Verification items for the finished model (mm, model axes). A direction names the side the tool comes from. Round coordinates to 2 decimals unless told otherwise and drop trailing zeros. Order: outer loops, then holes, each group sorted by start corner. A loop starts at its lowest first (then second) coordinate and runs counter-clockwise, first axis right, second up. Notation, with made-up numbers: (87, 42.5) -> (130, 42.5) arc R30 ccw to (130, 71.5) -> close; hole circle Ø10 at (26, 61). An arc over 180 degrees is marked (long way). Return JSON: item names as keys, results as strings. Group by question number.
1) Tool access check on faces 1 (the flat face through (-5.4, -3.2, 0)), 2 (the flat face through (5.4, -3.2, 0)), 3 (the flat face through (-5.4, 3, 0)). Record the directions out of +Z, -Z, +X, -X, +Y, -Y that give a thin tool (end or side, any length) a straight path to the whole face; none if there is none.
2) Depth check by flat-ended pin: pin 1 (2 mm diameter, centred on x = 2, z = -9.5, fed in from +Y); pin 2 (1 mm diameter, centred on x = 3.5, z = 4, fed in from +Y); pin 3 (2.5 mm diameter, centred on x = -2, y = -1, fed in from -Z). Enter the tip coordinate at first touch or a pass-through.
3) Section check A-A on z = 3. Enter the section's corners in (x, y), plus the area to 3 significant figures.
4) Section check D-D on z = -8.75. Enter the section's corners in (x, y), plus the area to 3 significant figures.
5) Scan lines: L1, parallel to Y at x = 0, z = -8.5; L2, parallel to Y at x = -2.75, z = -2; L3, parallel to Z at x = -2.25, y = 0.75. Record each from-to range of solid material in increasing order.
6) Draft check along Y on faces 4 (the flat face through (-2.96, 5.22, 2.96)), 5 (the flat face through (2, 0, 0)), 6 (the cylindrical face through (-6, 0, -6)). Enter one of: pulls with the +Y half, pulls with the -Y half, needs draft (parallel to the pull), parting line crosses it, or undercut.
7) Section check B-B on x = 2.25. Enter the section's corners in (y, z), plus the area to 3 significant figures.
8) Section check C-C on y = -3.25. Enter the section's corners in (x, z), plus the area to 3 significant figures.
```python
from build123d import *

# Parameters (mm, degrees)
SHAFT_SOCKET_START = -12
PROFILE_1_R        = 6
PROFILE_1_R_2      = 4
SHAFT_SOCKET_DEPTH = 12
PROFILE_2_R        = 1.65
DRIVE_HEX_DEPTH    = 6


with BuildPart() as part:
    # Profile_1 → Shaft_socket (new body)
    with BuildSketch(Plane.XY.offset(SHAFT_SOCKET_START)):
        Circle(PROFILE_1_R)
        Circle(PROFILE_1_R_2, mode=Mode.SUBTRACT)
    extrude(amount=SHAFT_SOCKET_DEPTH)

    # Profile_2 → Drive_hex (add)
    with BuildSketch(Plane.XY):
        Polygon((6, 3.464101615), (0, 6.92820323), (-6, 3.464101615), (-6, -3.464101615), (0, -6.92820323), (6, -3.464101615), align=None)
        Circle(PROFILE_2_R, mode=Mode.SUBTRACT)
    extrude(amount=DRIVE_HEX_DEPTH)


solid = part.part
```
Check result:
{
 "1": {"face 1": "-Z, -X, -Y", "face 2": "-Z, +X, -Y", "face 3": "-Z, -X, +Y"},
 "2": {"pin 1": "y = 5.92", "pin 2": "y = 5.2", "pin 3": "z = 0"},
 "3": {"outline": "(-6, -3.46) -> (0, -6.93) -> (6, -3.46) -> (6, 3.46) -> (0, 6.93) -> (-6, 3.46) -> close; hole circle Ø3.3 at (0, 0)", "area": "116 mm^2"},
 "4": {"outline": "circle Ø12 at (0, 0); hole circle Ø8 at (0, 0)", "area": "62.8 mm^2"},
 "5": {"L1": "-6 to -4, 4 to 6", "L2": "-5.33 to -2.9, 2.9 to 5.33", "L3": "0 to 6"},
 "6": {"face 4": "pulls with the +Y half", "face 5": "undercut", "face 6": "parting line crosses it"},
 "7": {"outline": "(-5.63, 0) -> (-5.56, 0) -> (-5.56, -12) -> (-3.31, -12) -> (-3.31, 0) -> (3.31, 0) -> (3.31, -12) -> (5.56, -12) -> (5.56, 0) -> (5.63, 0) -> (5.63, 6) -> (-5.63, 6) -> close", "area": "122 mm^2"},
 "8": {"outline": "(-6, 0) -> (-5.04, 0) -> (-5.04, -12) -> (-2.33, -12) -> (-2.33, 0) -> (2.33, 0) -> (2.33, -12) -> (5.04, -12) -> (5.04, 0) -> (6, 0) -> (6, 6) -> (-6, 6) -> close", "area": "137 mm^2"}
}
